from build123d import *

# Parameters (mm, degrees)
F1_DEPTH = 5
F2_R     = 1


with BuildPart() as f1:
    # F0 (on Top) → F1 (new body)
    with BuildSketch(Plane.XY):
        with BuildLine():
            ThreePointArc((-38.5927113062, 7.2194887325), (-35.5927113062, 10.2194887325), (-32.5927113062, 7.2194887325))
            ThreePointArc((-32.5927113062, 7.2194887325), (-29.5927113062, 4.2194887325), (-26.5927113062, 7.2194887325))
            ThreePointArc((-26.5927113062, 7.2194887325), (-23.5927113062, 10.2194887325), (-20.5927113062, 7.2194887325))
            ThreePointArc((-20.5927113062, 7.2194887325), (-17.5927113062, 4.2194887325), (-14.5927113062, 7.2194887325))
            ThreePointArc((-14.5927113062, 7.2194887325), (-11.5927113062, 10.2194887325), (-8.5927113062, 7.2194887325))
            ThreePointArc((-8.5927113062, 7.2194887325), (-5.5927113062, 4.2194887325), (-2.5927113062, 7.2194887325))
            ThreePointArc((-2.5927113062, 7.2194887325), (0.4072886938, 10.2194887325), (3.4072886938, 7.2194887325))
            ThreePointArc((3.4072886938, 7.2194887325), (6.4072886938, 4.2194887325), (9.4072886938, 7.2194887325))
            ThreePointArc((9.4072886938, 7.2194887325), (12.4072886938, 10.2194887325), (15.4072886938, 7.2194887325))
            ThreePointArc((15.4072886938, 7.2194887325), (18.4072886938, 4.2194887325), (21.4072886938, 7.2194887325))
            Line((21.4072886938, 7.2194887325), (23.1027154343, 7.2194887325))
            ThreePointArc((23.1027154343, 7.2194887325), (24.5169289967, 7.8052751701), (25.1027154343, 9.2194887325))
            Line((25.1027154343, 9.2194887325), (25.1027154343, 10.2194887325))
            ThreePointArc((25.1027154343, 10.2194887325), (24.5169289967, 11.6337022949), (23.1027154343, 12.2194887325))
            Line((23.1027154343, 12.2194887325), (-51.9450229577, 12.2194887325))
            ThreePointArc((-51.9450229577, 12.2194887325), (-90.0488899479, 3.7194887325), (-51.9450229577, -4.7805112675))
            Line((-51.9450229577, -4.7805112675), (23.0392886417, -4.7805112675))
            ThreePointArc((23.0392886417, -4.7805112675), (24.4535022041, -4.1947248299), (25.0392886417, -2.7805112675))
            Line((25.0392886417, -2.7805112675), (25.0392886417, -1.7805112675))
            ThreePointArc((25.0392886417, -1.7805112675), (24.4535022041, -0.3662977051), (23.0392886417, 0.2194887325))
            Line((23.0392886417, 0.2194887325), (21.4072886938, 0.2194887325))
            ThreePointArc((21.4072886938, 0.2194887325), (18.4072886938, -2.7805112675), (15.4072886938, 0.2194887325))
            ThreePointArc((15.4072886938, 0.2194887325), (12.4072886938, 3.2194887325), (9.4072886938, 0.2194887325))
            ThreePointArc((9.4072886938, 0.2194887325), (6.4072886938, -2.7805112675), (3.4072886938, 0.2194887325))
            ThreePointArc((3.4072886938, 0.2194887325), (0.4072886938, 3.2194887325), (-2.5927113062, 0.2194887325))
            ThreePointArc((-2.5927113062, 0.2194887325), (-5.5927113062, -2.7805112675), (-8.5927113062, 0.2194887325))
            ThreePointArc((-8.5927113062, 0.2194887325), (-11.5927113062, 3.2194887325), (-14.5927113062, 0.2194887325))
            ThreePointArc((-14.5927113062, 0.2194887325), (-17.5927113062, -2.7805112675), (-20.5927113062, 0.2194887325))
            ThreePointArc((-20.5927113062, 0.2194887325), (-23.5927113062, 3.2194887325), (-26.5927113062, 0.2194887325))
            ThreePointArc((-26.5927113062, 0.2194887325), (-29.5927113062, -2.7805112675), (-32.5927113062, 0.2194887325))
            ThreePointArc((-32.5927113062, 0.2194887325), (-35.5927113062, 3.2194887325), (-38.5927113062, 0.2194887325))
            Line((-38.5927113062, 0.2194887325), (-55.4629378021, 0.2194887325))
            ThreePointArc((-55.4629378021, 0.2194887325), (-85.0488899479, 3.7194887325), (-55.4629378021, 7.2194887325))
            Line((-55.4629378021, 7.2194887325), (-38.5927113062, 7.2194887325))
        make_face()
    extrude(amount=F1_DEPTH)

    # F2
    f2_edges = [f1.edges().sort_by_distance(p)[0] for p in [
        (-55.462938, 7.219489, 2.5),
        (-38.592711, 7.219489, 2.5),
        (-38.592711, 0.219489, 2.5),
        (-55.462938, 0.219489, 2.5),
        (21.407289, 0.219489, 2.5),
        (21.407289, 7.219489, 2.5),
    ]]
    fillet(f2_edges, radius=F2_R)


solid = f1.part
Work out the finished part from the listing and answer in its coordinate system (mm). A direction names the side the tool comes from. Round coordinates to 2 decimals unless told otherwise and drop trailing zeros. Write each loop counter-clockwise with the first axis right and the second up, starting at its lowest first coordinate (ties: lowest second). Pieces come first, ordered by that corner, then holes. Notation, with made-up numbers: (66.5, -10.5) -> (95.5, -10.5) arc R36 ccw to (95.5, 26.5) -> close; hole circle Ø11 at (71, -17). An arc over 180 degrees is marked (long way). Answer as CSV lines item,"result". Start each with the question number.
(1) The part is cut by section C-C, the plane y = 20. Give the vertices of the cut face in (x, z), then the cut area to 3 significant figures.
(2) The mould has two halves that part along X. Classify faces 1 (the flat face through (-37, 2, 0)), 2 (the flat face through (-47, 7.219, 2)), 3 (the flat face through (-47, 0.219, 2)), 4 (the cylindrical face through (24.53, 11.62, 2.46)): +X half, -X half, draft (parallel to the pull), parting line (faces both ways), or undercut.
(3) The part is cut by section B-B, the plane y = 14. Give the vertices of the cut face in (x, z), then the cut area to 3 significant figures.
(4) The part is cut by section A-A, the plane x = -12. Give the vertices of the cut face in (y, z).
(5) Each of these flat-tipped pins is pushed along its axis until it touches: pin 1 (2.5 mm diameter, centred on x = -5, z = 2.5, fed in from -Y); pin 2 (2.5 mm diameter, centred on x = -21.5, z = 2, fed in from +Y); pin 3 (6 mm diameter, centred on x = -49.5, y = 12.5, fed in from +Z); pin 4 (0.5 mm diameter, centred on y = -2.5, z = 3.5, fed in from +X). Where does it stop, or does it pass through?
(6) A tool of negligible diameter and unlimited length cuts with its end or side. For faces 5 (the flat face through (-14, 12.219, 2)), 6 (the cylindrical face through (24.469, -0.382, 2.465)), 7 (the flat face through (-15, -4.781, 2)), from which of +Z, -Z, +X, -X, +Y, -Y can it reach the whole face along a straight path? Write none if from no direction.
(7) Find the intervals of material crossed by probe 1 along Y at (x, z) = (-40, 4.4); probe 2 along X at (y, z) = (6.5, 2.4); probe 3 along Y at (x, z) = (-17.5, 1.4), in increasing order.
Output values:
1,outline,"(-81.67, 0) -> (-58.43, 0) -> (-58.43, 5) -> (-81.67, 5) -> close"
1,area,"116 mm²"
2,face 1,"draft"
2,face 2,"undercut"
2,face 3,"undercut"
2,face 4,"+X half"
3,outline,"(-87.2, 0) -> (-80.97, 0) -> (-80.97, 5) -> (-87.2, 5) -> close; (-59.13, 0) -> (-52.89, 0) -> (-52.89, 5) -> (-59.13, 5) -> close"
3,area,"62.3 mm²"
4,outline,"(-4.78, 0) -> (3.19, 0) -> (3.19, 5) -> (-4.78, 5) -> close; (10.19, 0) -> (12.22, 0) -> (12.22, 5) -> (10.19, 5) -> close"
5,pin 1,"stops at y = -4.78"
5,pin 2,"stops at y = 12.22"
5,pin 3,"stops at z = 5"
5,pin 4,"stops at x = 25.04"
6,face 5,"+Z, -Z, +X, +Y"
6,face 6,"+Z, -Z, +X"
6,face 7,"+Z, -Z, +X, -Y"
7,probe 1,"y = -4.78 to 0.22, 7.22 to 12.22"
7,probe 2,"x = -89.85 to -84.79, -32.51 to -26.68, -20.51 to -14.68, -8.51 to -2.68, 3.49 to 9.32, 15.49 to 21.32"
7,probe 3,"y = -4.78 to -2.78, 4.22 to 12.22"
